Read the model definition and answer for the solid it produces. Units are mm, in the model's axes. Face numbers are marked on the shaded views. A direction names the side the tool comes from. Give positions to 0.01 mm unless a question says otherwise; leave off trailing zeros. Write each loop counter-clockwise with the first axis right and the second up, starting at its lowest first coordinate (ties: lowest second). Pieces come first, ordered by that corner, then holes. Notation, with made-up numbers: M 9.5,35 L 13.5,35 A11 cw 13.5,55 Z; hole C 24,29.5 d3. An arc over 180 degrees is marked long. Put each result on its own line as item: value.
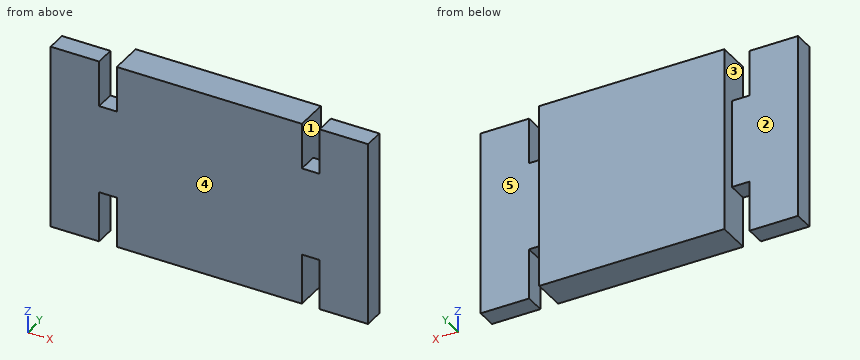
from build123d import *

# Parameters (mm, degrees)
EXTRUDE_1_DEPTH = 3
SKETCH_3_W      = 28
SKETCH_3_H      = 28
EXTRUDE_2_DEPTH = 1
SKETCH_4_W      = 28
SKETCH_4_H      = 28
EXTRUDE_3_DEPTH = 1


with BuildPart() as part:
    # 草图2 → 凸台-拉伸1 (new body)
    with BuildSketch(Plane(origin=(0, 0, 0), x_dir=(1, 0, 0), z_dir=(0, 1, 0))):
        Polygon((0, 9.283892138), (-2.678979425, 9.283892138), (-2.678979425, 16.936687797), (-10, 16.936687797), (-10, -11.063312203), (-2.678979425, -11.063312203), (-2.678979425, -4.12513502), (0, -4.12513502), (0, -11.063312203), (28, -11.063312203), (28, -4.12513502), (30.678979425, -4.12513502), (30.678979425, -11.063312203), (38, -11.063312203), (38, 16.936687797), (30.678979425, 16.936687797), (30.678979425, 9.283892138), (28, 9.283892138), (28, 16.936687797), (0, 16.936687797), align=None)
    extrude(amount=EXTRUDE_1_DEPTH)

    # 草图3 → 凸台-拉伸2 (add)
    with BuildSketch(Plane(origin=(0, 3, 0), x_dir=(1, 0, 0), z_dir=(0, 1, 0))):
        with Locations((14, 2.936687797)):
            Rectangle(SKETCH_3_W, SKETCH_3_H)
    extrude(amount=EXTRUDE_2_DEPTH)

    # 草图4 → 凸台-拉伸3 (add)
    with BuildSketch(Plane(origin=(0, 4, 0), x_dir=(1, 0, 0), z_dir=(0, 1, 0))):
        with Locations((14, 2.936687797)):
            Rectangle(SKETCH_4_W, SKETCH_4_H)
    extrude(amount=EXTRUDE_3_DEPTH)


solid = part.part
(1) Section B-B on z = -14.75 is taken. Determine the outline of the cut face in (x, y).
Result:
outline: M -10,0 L -2.68,0 L -2.68,3 L -10,3 Z; M 0,0 L 28,0 L 28,5 L 0,5 Z; M 30.68,0 L 38,0 L 38,3 L 30.68,3 Z
(2) Section C-C on y = 2.3 is taken. Determine the outline of the cut face in (x, z).
Result:
outline: M -10,-16.94 L -2.68,-16.94 L -2.68,-9.28 L 0,-9.28 L 0,-16.94 L 28,-16.94 L 28,-9.28 L 30.68,-9.28 L 30.68,-16.94 L 38,-16.94 L 38,11.06 L 30.68,11.06 L 30.68,4.13 L 28,4.13 L 28,11.06 L 0,11.06 L 0,4.13 L -2.68,4.13 L -2.68,11.06 L -10,11.06 Z
(3) Which of the six approach directions +Z, -Z, +X, -X, +Y, -Y give full straight-line access (tool end or side, diameter ignored) to the marked faces 4 and 5?
Result:
face 4: +Z, -Z, +X, -X, -Y
face 5: +Z, -Z, +X, +Y
(4) Given pin 1 Ø1.5 at (y, z) = (4, 6.5) entering from +X; pin 2 Ø5 at (x, z) = (-5.5, -7) entering from +Y; pin 3 Ø0.8 at (x, y) = (-2, 2) entering from +Z, each flat-ended and moving along its own axis, determine where each tip first touches the part or whether it passes through.
Result:
pin 1: stops at x = 28
pin 2: stops at y = 3
pin 3: stops at z = 4.13
(5) Straight lines are drawn through the part: line 1 along X through (y, z) = (0.9, -13.75); line 2 along Y through (x, z) = (35, -7.5); line 3 along X through (y, z) = (3.95, -2.5). For each, find the intervals that lie inside material, in ascending order. Write a range as from..to.
Result:
line 1: x = -10..-2.68, 0..28, 30.68..38
line 2: y = 0..3
line 3: x = 0..28
(6) For a pull along X with two mould halves and no side action, classify the marked faces 1, 2 and 3 as +X half, -X half, draft (parallel to the pull), parting line (faces both ways), or undercut.
Result:
face 1: undercut
face 2: draft
face 3: undercut
(7) Section A-A on z = -2.5 is taken. Determine the outline of the cut face in (x, y).
Result:
outline: M -10,0 L 38,0 L 38,3 L 28,3 L 28,5 L 0,5 L 0,3 L -10,3 Z
(8) Section D-D on x = -4 is taken. Determine the outline of the cut face in (y, z), and give its area (3 significant figures).
Result:
outline: M 0,-16.94 L 3,-16.94 L 3,11.06 L 0,11.06 Z
area: 84.0 mm²
